Design review of the part built by this model. Coordinates are the model's own, in mm. Coordinates: 2 decimals unless noted, no trailing zeros. Loops run counter-clockwise (first coordinate to the right, second up) from the corner with the lowest first, then second, coordinate; pieces in that order, holes last. Notation, with made-up numbers: (36.25, -11) -> (41.25, -11) arc R8 ccw to (41.25, 3) -> close; hole circle Ø5 at (11.5, 0). An arc over 180 degrees is marked (long way). Use CSV: the item, a comma, the result in double quotes.
```python
from build123d import *

# Parameters (mm, degrees)
SKETCH2_R           = 85.09
SKETCH2_R_2         = 12.7
SKETCH2_W           = 104.14
SKETCH2_H           = 104.14
BOSS_EXTRUDE1_DEPTH = 2.54


with BuildPart() as part:
    # Sketch2 → Boss-Extrude1 (new body)
    with BuildSketch(Plane.YZ):
        with Locations(Location((0, 0, 0), (0, 0, 270))):
            Circle(SKETCH2_R)
        with Locations(Location((0, 67.31, 0), (0, 0, 270))):
            Circle(SKETCH2_R_2, mode=Mode.SUBTRACT)
        with Locations(Location((67.31, 0, 0), (0, 0, 270))):
            Circle(SKETCH2_R_2, mode=Mode.SUBTRACT)
        with Locations(Location((0, -67.31, 0), (0, 0, 270))):
            Circle(SKETCH2_R_2, mode=Mode.SUBTRACT)
        with Locations(Location((-67.31, 0, 0), (0, 0, 270))):
            Circle(SKETCH2_R_2, mode=Mode.SUBTRACT)
        Rectangle(SKETCH2_W, SKETCH2_H, mode=Mode.SUBTRACT)
    extrude(amount=BOSS_EXTRUDE1_DEPTH)


solid = part.part
```
Item 1: Clearance check with flat-ended pins moving along their axes: pin 1 (0.8 mm diameter, centred on x = 1.5, z = 2, fed in from -Y); pin 2 (1 mm diameter, centred on x = 2, z = -66.5, fed in from -Y); pin 3 (0.8 mm diameter, centred on x = 1.5, z = -23, fed in from +Y). State where each tip first meets the part, or that it passes through.
Checked values:
pin 1,"y = -85.07"
pin 2,"y = -53.71"
pin 3,"y = 82.03"
Item 2: Add section C-C (y = -71). Give the boundary of the cut face in (x, z).
Checked values:
outline,"(0, -46.9) -> (2.54, -46.9) -> (2.54, -12.15) -> (0, -12.15) -> close; (0, 12.15) -> (2.54, 12.15) -> (2.54, 46.9) -> (0, 46.9) -> close"
Item 3: Add section B-B (x = 0.4). Give the boundary of the cut face in (y, z).
Checked values:
outline,"circle Ø170.18 at (0, 0); hole circle Ø25.4 at (-67.31, 0); hole (-52.07, -52.07) -> (52.07, -52.07) -> (52.07, 52.07) -> (-52.07, 52.07) -> close; hole circle Ø25.4 at (0, -67.31); hole circle Ø25.4 at (0, 67.31); hole circle Ø25.4 at (67.31, 0)"
Item 4: Add section D-D (z = -60). Give the boundary of the cut face in (x, y).
Checked values:
outline,"(0, -60.33) -> (2.54, -60.33) -> (2.54, -10.39) -> (0, -10.39) -> close; (0, 10.39) -> (2.54, 10.39) -> (2.54, 60.33) -> (0, 60.33) -> close"
Item 5: Add section A-A (z = 0). Give the boundary of the cut face in (x, y), then the cut area to 3 significant figures.
Checked values:
outline,"(0, -85.09) -> (2.54, -85.09) -> (2.54, -80.01) -> (0, -80.01) -> close; (0, -54.61) -> (2.54, -54.61) -> (2.54, -52.07) -> (0, -52.07) -> close; (0, 52.07) -> (2.54, 52.07) -> (2.54, 54.61) -> (0, 54.61) -> close; (0, 80.01) -> (2.54, 80.01) -> (2.54, 85.09) -> (0, 85.09) -> close"
area,"38.7 mm^2"
Item 6: To check wall thickness, follow line 1 along Y through (x, z) = (1, 0); line 2 along Z through (x, y) = (1.05, 29); line 3 along Y through (x, z) = (1.85, -67.31). State the ranges of each line that lie inside material, in increasing order.
Checked values:
line 1,"-85.09 to -80.01, -54.61 to -52.07, 52.07 to 54.61, 80.01 to 85.09"
line 2,"-80 to -52.07, 52.07 to 80"
line 3,"-52.05 to -12.7, 12.7 to 52.05"
Item 7: Draft analysis for pull direction Y (two halves, no side actions). For faces 1 (the face through (1.252, -83.067, 18.446)), 2 (the face through (1.252, 79.902, 1.653)), 3 (the face through (0, -56, -18)), state which applies: pulls with the +Y half, pulls with the -Y half, needs draft (parallel to the pull), parting line crosses it, or undercut.
Checked values:
face 1,"parting line crosses it"
face 2,"undercut"
face 3,"needs draft"
